```python
from build123d import *

# Parameters (mm, degrees)
BOSS_EXTRUDE1_DEPTH = 9.525
RIB1_REACH          = 156.901
SKETCH3_WALL_W      = 425.12827586
SKETCH3_WALL_H      = 9.525
BOSS_EXTRUDE2_DEPTH = 12.7
SKETCH4_W           = 31.75
SKETCH4_H           = 15.875
BOSS_EXTRUDE3_DEPTH = 41.275
SKETCH10_W          = 41.275
SKETCH10_H          = 68.618379108
BOSS_EXTRUDE4_DEPTH = 6.35
CUT_EXTRUDE5_START  = -67.495198541
CUT_EXTRUDE5_DEPTH  = 73.845198541
SKETCH14_R          = 7.540625
CUT_EXTRUDE6_DEPTH  = 6.35
SKETCH15_R          = 5.159375
CUT_EXTRUDE7_DEPTH  = 156.055766211


with BuildPart() as part:
    # Sketch1 → Boss-Extrude1 (new body)
    with BuildSketch(Plane.XY):
        with BuildLine():
            ThreePointArc((-61.11875, 127), (-31.75, 97.63125), (-2.38125, 127))
            Line((-2.38125, 127), (-2.38125, 136.525))
            Line((-2.38125, 136.525), (9.525, 136.525))
            Line((9.525, 136.525), (9.525, 127))
            Line((9.525, 127), (9.525, 15.875))
            Line((9.525, 15.875), (31.75, 15.875))
            Line((31.75, 15.875), (31.75, 0))
            Line((31.75, 0), (0, 0))
            Line((0, 0), (0, 15.875))
            Line((0, 15.875), (-64.77, 102.235))
            ThreePointArc((-64.77, 102.235), (-70.906903127, 113.947698958), (-73.025, 127))
            Line((-73.025, 127), (-73.025, 136.525))
            Line((-73.025, 136.525), (-61.11875, 136.525))
            Line((-61.11875, 136.525), (-61.11875, 127))
        make_face()
        with BuildLine():
            ThreePointArc((-73.025, 127), (-71.61858848, 116.317243913), (-67.495198541, 106.3625))
            Line((-67.495198541, 106.3625), (-57.184083577, 112.315625))
            ThreePointArc((-57.184083577, 112.315625), (-60.118034111, 119.398808169), (-61.11875, 127))
            Line((-61.11875, 127), (-61.11875, 136.525))
            Line((-61.11875, 136.525), (-73.025, 136.525))
            Line((-73.025, 136.525), (-73.025, 127))
        make_face()
        with BuildLine():
            Line((-6.315916423, 112.315625), (9.525, 103.169867639))
            Line((9.525, 103.169867639), (9.525, 127))
            Line((9.525, 127), (9.525, 136.525))
            Line((9.525, 136.525), (-2.38125, 136.525))
            Line((-2.38125, 136.525), (-2.38125, 127))
            ThreePointArc((-2.38125, 127), (-3.381965889, 119.398808169), (-6.315916423, 112.315625))
        make_face()
    extrude(amount=BOSS_EXTRUDE1_DEPTH)

    # Sketch3 wall → Rib1 (add, up to next)
    with BuildSketch(Plane(origin=(20.6375, 71.4375, 4.7625), x_dir=(-0.196116135138, 0.980580675691, 0), z_dir=(-0.980580675691, -0.196116135138, 0)), mode=Mode.PRIVATE) as rib1_sk1:
        Rectangle(SKETCH3_WALL_W, SKETCH3_WALL_H)
    rib1_tool1 = extrude(rib1_sk1.sketch, amount=RIB1_REACH, mode=Mode.PRIVATE) - part.part
    add(rib1_tool1.solids().sort_by_distance((20.6375, 71.4375, 4.7625))[0])

    # Sketch1_3 → Boss-Extrude2 (add)
    with BuildSketch(Plane.XY):
        with BuildLine():
            ThreePointArc((-73.025, 127), (-71.61858848, 116.317243913), (-67.495198541, 106.3625))
            Line((-67.495198541, 106.3625), (-57.184083577, 112.315625))
            ThreePointArc((-57.184083577, 112.315625), (-60.118034111, 119.398808169), (-61.11875, 127))
            Line((-61.11875, 127), (-61.11875, 136.525))
            Line((-61.11875, 136.525), (-73.025, 136.525))
            Line((-73.025, 136.525), (-73.025, 127))
        make_face()
        with BuildLine():
            Line((-6.315916423, 112.315625), (9.525, 103.169867639))
            Line((9.525, 103.169867639), (9.525, 127))
            Line((9.525, 127), (9.525, 136.525))
            Line((9.525, 136.525), (-2.38125, 136.525))
            Line((-2.38125, 136.525), (-2.38125, 127))
            ThreePointArc((-2.38125, 127), (-3.381965889, 119.398808169), (-6.315916423, 112.315625))
        make_face()
    extrude(amount=BOSS_EXTRUDE2_DEPTH)

    # Sketch4 → Boss-Extrude3 (add)
    with BuildSketch(Plane.XY.offset(9.525)):
        with Locations((15.875, 7.9375)):
            Rectangle(SKETCH4_W, SKETCH4_H)
    extrude(amount=BOSS_EXTRUDE3_DEPTH)

    # Sketch10 → Boss-Extrude4 (add, along a direction that is not the sketch's normal)
    with BuildSketch(Plane(origin=(4.193396226, 1.198113208, 0), x_dir=(0, 0, -1), z_dir=(0.9615239476408233, 0.2747211278973781, 0))):
        with Locations((-30.1625, 49.573382223)):
            Rectangle(SKETCH10_W, SKETCH10_H)
    extrude(amount=BOSS_EXTRUDE4_DEPTH, dir=(1, 0, 0))

    # Cut-Extrude5: read off the stored shape, not the designer's step
    # Cut-Extrude5 outline → Cut-Extrude5 (cut)
    with BuildSketch(Plane.YZ.offset(CUT_EXTRUDE5_START)):
        Polygon((55.561900939, 9.525), (81.85321476, 9.525), (81.85321476, 50.8), (15.875, 50.8), align=None)
    extrude(amount=CUT_EXTRUDE5_DEPTH, mode=Mode.SUBTRACT)

    # Sketch13 → Loft2 section 0
    with BuildSketch(Plane(origin=(10.064150943, 2.875471698, 0), x_dir=(0, 0, -1), z_dir=(0.9615239476408232, 0.27472112789737807, 0))):
        with BuildLine():
            Line((-18.177760419, 46.141953088), (-8.652760419, 83.010332195))
            Line((-8.652760419, 83.010332195), (-9.525, 54.794713507))
            Line((-9.525, 54.794713507), (-18.177760419, 46.141953088))
        make_face()
    # Sketch12 → Loft2 section 1
    with BuildSketch(Plane(origin=(4.193396226, 1.198113208, 0), x_dir=(0, 0, -1), z_dir=(0.9615239476408233, 0.2747211278973781, 0))):
        with BuildLine():
            Line((-19.05, 47.014192669), (-9.525, 83.882571777))
            Line((-9.525, 83.882571777), (-9.525, 56.539192669))
            Line((-9.525, 56.539192669), (-19.05, 47.014192669))
        make_face()
    loft()

    # Sketch14 → Cut-Extrude6 (cut)
    with BuildSketch(Plane(origin=(0, 15.875, 0), x_dir=(1, 0, 0), z_dir=(0, 1, 0))):
        with Locations(Location((15.875, -41.275, 0), (0, 0, 270))):
            Circle(SKETCH14_R)
        with Locations(Location((15.875, -22.225, 0), (0, 0, 270))):
            Circle(SKETCH14_R)
    extrude(amount=-CUT_EXTRUDE6_DEPTH, mode=Mode.SUBTRACT)

    # Sketch15 → Cut-Extrude7 (cut, through all)
    with BuildSketch(Plane(origin=(0, 9.525, 0), x_dir=(1, 0, 0), z_dir=(0, 1, 0))):
        with Locations(Location((15.875, -22.225, 0), (0, 0, 270))):
            Circle(SKETCH15_R)
        with Locations(Location((15.875, -41.275, 0), (0, 0, 270))):
            Circle(SKETCH15_R)
    extrude(amount=-CUT_EXTRUDE7_DEPTH, mode=Mode.SUBTRACT)


solid = part.part
```
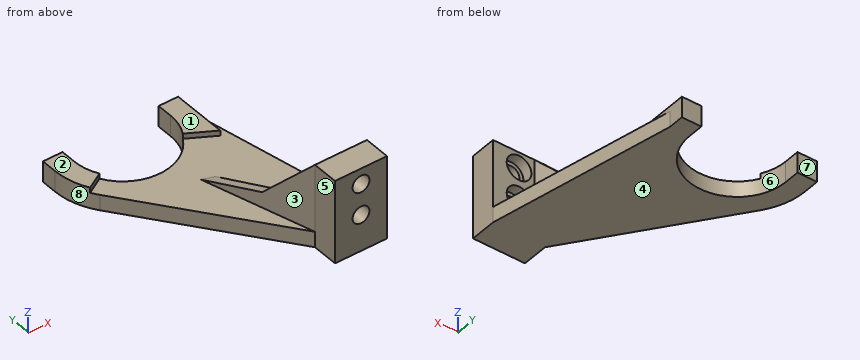
The listing builds one solid part. Answer for the finished solid, in the listing's coordinates (mm). Face numbers are marked on the shaded views. A direction names the side the tool comes from. Round coordinates to 2 decimals unless told otherwise and drop trailing zeros. Loops run counter-clockwise (first coordinate to the right, second up) from the corner with the lowest first, then second, coordinate; pieces in that order, holes last.
Q1. Find the intervals of material crossed by line 1 (X direction, y = 131.5, z = 3.5) (3 decimals); line 2 (Y direction, x = 10, z = 24.5) (3 decimals), in increasing order.
Q2. Given pin 1 Ø3 at (y, z) = (132.5, 6) entering from +X (3 decimals); pin 2 Ø16.5 at (x, z) = (15.875, 41.275) entering from +Y (3 decimals); pin 3 Ø12.5 at (x, y) = (-62.5, 121.5) entering from +Z, each flat-ended and moving along its own axis, determine where each tip first touches the part or whether it passes through.
Q3. Which of the six approach directions +Z, -Z, +X, -X, +Y, -Y give full straight-line access (tool end or side, diameter ignored) to the marked faces 1, 2, 3, 4 and 5?
Q4. Section B-B, the plane y = 36 is taken. Determine the outline of the cut face in (x, z) (3 decimals), then the cut area to 3 significant figures.
Q5. Section A-A, the plane z = 38.5 is taken. Determine the outline of the cut face in (x, y) (3 decimals).
Q6. For a pull along X with two mould halves and no side action, classify the marked faces 6, 7 and 8 as released by +X, released by -X, zero draft, split by the parting line, or undercut.
Q7. Section D-D, the plane z = 25 is taken. Determine the outline of the cut face in (x, y) (3 decimals).
Completed:
1. line 1: x = -73.025 to -61.119, -2.381 to 9.525
1. line 2: y = 0 to 9.525
2. pin 1: stops at x = 9.525
2. pin 2: stops at y = 15.875
2. pin 3: stops at z = 12.7
3. face 1: +Z, +X, -X, +Y
3. face 2: +Z, +X, -X, +Y, -Y
3. face 3: +Z, -X, -Y
3. face 4: -Z, +X, -X, +Y, -Y
3. face 5: +Z, -Z, -X, -Y
4. outline: (-15.094, 0) - (27.725, 0) - (27.725, 9.525) - (0.6, 9.525) - (0.6, 29.87) - (-5.75, 29.87) - (-5.75, 9.525) - (-15.094, 9.525) - close
4. area: 537 mm2
5. outline: (-3.379, 27.702) - (0, 15.875) - (0, 0) - (11.525, 0) - (11.525, 9.525) - (8.864, 9.525) - (8.864, 15.875) - (6.35, 15.875) - (2.971, 27.702) - close; (20.225, 0) - (31.75, 0) - (31.75, 15.875) - (22.886, 15.875) - (22.886, 9.525) - (20.225, 9.525) - close
6. face 6: undercut
6. face 7: zero draft
6. face 8: released by -X
7. outline: (-7.088, 40.682) - (0, 15.875) - (0, 0) - (11.525, 0) - (11.525, 9.525) - (8.864, 9.525) - (8.864, 15.875) - (6.35, 15.875) - (-0.738, 40.682) - close; (20.225, 0) - (31.75, 0) - (31.75, 15.875) - (22.886, 15.875) - (22.886, 9.525) - (20.225, 9.525) - close
